```python
from build123d import *

# Parameters (mm, degrees)
F1_DEPTH = 25.4
F2_R     = 0.79374


# Not quite as in the source:
# - a fillet or chamfer is up to 0.001 mm smaller than in the source, because OpenCascade refuses the exact size
# - a feature names something its author has since deleted; it is built from what else it names


with BuildPart() as f1:
    # F0 (on Top) → F1 (new body)
    with BuildSketch(Plane.XY):
        with BuildLine():
            ThreePointArc((2.2450640303, -0.79375), (2.3469565702, -0.4026740868), (2.38125, 0))
            ThreePointArc((2.38125, 0), (2.3469565702, 0.4026740868), (2.2450640303, 0.79375))
            ThreePointArc((2.2450640303, 0.79375), (-2.38125, 0), (2.2450640303, -0.79375))
        make_face()
        with BuildLine():
            ThreePointArc((2.2450640303, 0.79375), (2.3469565702, 0.4026740868), (2.38125, 0))
            ThreePointArc((2.38125, 0), (2.3469565702, -0.4026740868), (2.2450640303, -0.79375))
            Line((2.2450640303, -0.79375), (33.9950640303, -0.79375))
            Line((33.9950640303, -0.79375), (33.9950640303, 0))
            Line((33.9950640303, 0), (33.9950640303, 0.79375))
            Line((33.9950640303, 0.79375), (2.2450640303, 0.79375))
        make_face()
    extrude(amount=F1_DEPTH)

    # F2 (radius 0.79375 in the source; OpenCascade refuses exactly that, so slightly less here)
    f2_edges = [f1.edges().sort_by_distance(p)[0] for p in [
        (-2.38125, 0, 25.4),
        (18.120064, -0.79375, 25.4),
        (33.995064, 0, 25.4),
        (18.120064, 0.79375, 25.4),
        (-2.38125, 0, 0),
        (18.120064, -0.79375, 0),
        (33.995064, 0, 0),
        (18.120064, 0.79375, 0),
        (33.995064, 0.79375, 12.7),
        (2.245064, 0.79375, 12.7),
        (2.245064, -0.79375, 12.7),
        (33.995064, -0.79375, 12.7),
    ]]
    fillet(f2_edges, radius=F2_R)


solid = f1.part
```
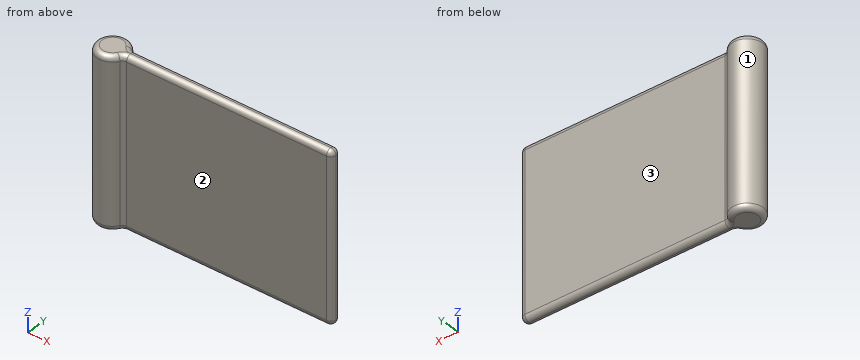
The model under review builds one solid part; all positions refer to its coordinate system, in mm. Face numbers are marked on the shaded views. A direction names the side the tool comes from. Round coordinates to 2 decimals unless told otherwise and drop trailing zeros.
1) Wall thickness on line 1 along Y through (x, z) = (10, 15.75); line 2 along X through (y, z) = (-1.25, 18.5); line 3 along X through (y, z) = (2, 17): over which ranges is each line inside the solid? List them lowest first.
Values follow:
line 1: y = -0.79 to 0.79
line 2: x = -2.03 to 2.03
line 3: x = -1.29 to 1.29
2) Tool access review of the marked faces 1, 2 and 3: name each direction out of +Z, -Z, +X, -X, +Y, -Y from which nothing blocks a thin tool from reaching the whole face with its end or side.
Values follow:
face 1: +Z, -Z
face 2: +Z, -Z, +X, -Y
face 3: +Z, -Z, +X, +Y
3) Clearance check with flat-ended pins moving along their axes: P1, Ø2, axis at y = 2, z = 8, coming from the +X side; P2, Ø7, axis at x = 20, z = 16, coming from the +Y side; P3, Ø7, axis at x = 19.5, z = 13, coming from the -Y side. State where each tip first meets the part, or that it passes through.
Values follow:
P1: stops at x = 2.22
P2: stops at y = 0.79
P3: stops at y = -0.79
